```python
from build123d import *

# Parameters (mm, degrees)
SKETCH_W     = 12
SKETCH_H     = 9
SKETCH_R     = 1.7
PAD_DEPTH    = 2
SKETCH001_W  = 3.1
SKETCH001_H  = 4.7
PAD001_DEPTH = 2
SKETCH002_W  = 1.1
SKETCH002_H  = 5
POCKET_DEPTH = 4.001
CHAMFER_SIZE = 1.7


with BuildPart() as part:
    # Sketch → Pad (new body)
    with BuildSketch(Plane.XY):
        with Locations((-1.5, 0)):
            Rectangle(SKETCH_W, SKETCH_H)
        with Locations((-3, 0)):
            Circle(SKETCH_R, mode=Mode.SUBTRACT)
    extrude(amount=PAD_DEPTH)

    # Sketch001 → Pad001 (new body)
    with BuildSketch(Plane.XY.offset(2)):
        with Locations((1.75, 0)):
            Rectangle(SKETCH001_W, SKETCH001_H)
    extrude(amount=PAD001_DEPTH)

    # Sketch002 → Pocket (cut, through all)
    with BuildSketch(Plane.XY.offset(4)):
        with Locations((1.75, 4)):
            Rectangle(SKETCH002_W, SKETCH002_H)
        with Locations((1.75, -4)):
            Rectangle(SKETCH002_W, SKETCH002_H)
    extrude(amount=-POCKET_DEPTH, mode=Mode.SUBTRACT)

    # Chamfer
    chamfer_edges = [part.edges().sort_by_distance(p)[0] for p in [
        (-4.7, 0, 0),
    ]]
    chamfer(chamfer_edges, length=CHAMFER_SIZE)


solid = part.part
```
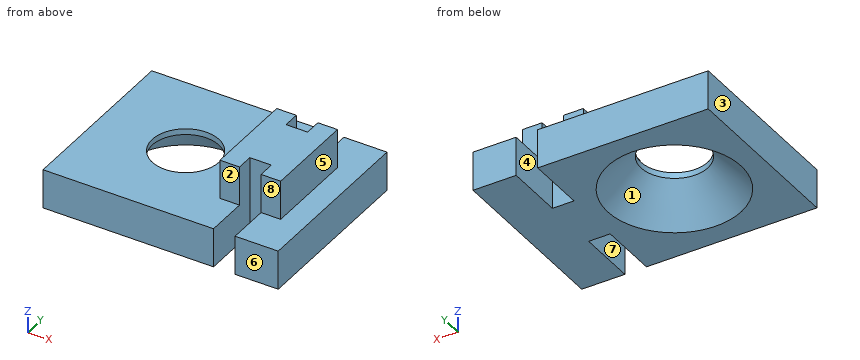
The model under review builds one solid part; all positions refer to its coordinate system, in mm. Face numbers are marked on the shaded views. A direction names the side the tool comes from. Coordinates: 2 decimals unless noted, no trailing zeros. Write each loop counter-clockwise with the first axis right and the second up, starting at its lowest first coordinate (ties: lowest second). Pieces come first, ordered by that corner, then holes. Notation, with made-up numbers: (60.25, -0.5) - (95.25, -0.5) arc R18 cw to (95.25, 14.5) - close; hole circle Ø11 at (-2, -14.5). An arc over 180 degrees is marked (long way). Write item = value, one per line.
(1) For P1, Ø0.5, axis at x = 0.5, z = 2.5, coming from the -Y side; P2, Ø4.5, axis at x = -4.5, y = -1.5, coming from the +Z side, all flat-tipped, find the tip position at first contact; note any pin that passes through.
Result sheet:
P1 = -2.35
P2 = 2
(2) Machinability: for the marked faces 4, 5, 6, 7 and 8, which of the approach directions +Z, -Z, +X, -X, +Y, -Y give a long, thin tool a straight path to every point of the face, cutting with its end or side? Answer none if there is none.
Result sheet:
face_4 = +Z, -Z, +Y
face_5 = +Z, +X, +Y, -Y
face_6 = +Z, -Z, +X, -X, -Y
face_7 = +Z, -Z, -Y
face_8 = +Z, +X, -X, -Y
(3) Consider section D-D, the plane x = 2.5. Give the boundary of the cut face in (y, z).
Result sheet:
outline = (-4.5, 0) - (4.5, 0) - (4.5, 2) - (2.35, 2) - (2.35, 4) - (-2.35, 4) - (-2.35, 2) - (-4.5, 2) - close
(4) For line 1 (X direction, y = 4, z = 0.8); line 2 (X direction, y = 2, z = 0.65); line 3 (X direction, y = 1.75, z = 0.3), list the stretches that pass through material, from the lowest coordinate up. Write a range as [from, to].
Result sheet:
line_1 = [-7.5, 1.2], [2.3, 4.5]
line_2 = [-7.5, -4.89], [-1.11, 1.2], [2.3, 4.5]
line_3 = [-7.5, -5.56], [-0.44, 1.2], [2.3, 4.5]
(5) Consider section B-B, the plane z = 0.9. Give the boundary of the cut face in (x, y).
Result sheet:
outline = (-7.5, -4.5) - (1.2, -4.5) - (1.2, -1.5) - (2.3, -1.5) - (2.3, -4.5) - (4.5, -4.5) - (4.5, 4.5) - (2.3, 4.5) - (2.3, 1.5) - (1.2, 1.5) - (1.2, 4.5) - (-7.5, 4.5) - close; hole circle Ø5 at (-3, 0)
(6) Consider section C-C, the plane y = 0. Give the boundary of the cut face in (x, z).
Result sheet:
outline = (-7.5, 0) - (-6.4, 0) - (-4.7, 1.7) - (-4.7, 2) - (-7.5, 2) - close; (-1.3, 1.7) - (0.4, 0) - (4.5, 0) - (4.5, 2) - (3.3, 2) - (3.3, 4) - (0.2, 4) - (0.2, 2) - (-1.3, 2) - close
(7) Consider section A-A, the plane x = -3. Give the boundary of the cut face in (y, z), then the cut area to 3 significant figures.
Result sheet:
outline = (-4.5, 0) - (-3.4, 0) - (-1.7, 1.7) - (-1.7, 2) - (-4.5, 2) - close; (1.7, 1.7) - (3.4, 0) - (4.5, 0) - (4.5, 2) - (1.7, 2) - close
area = 8.31 mm^2
(8) Mouldability with a two-part tool opening along X and no side actions: class the marked faces 1, 2 and 3 as pulls with the +X half, pulls with the -X half, needs draft (parallel to the pull), parting line crosses it, or undercut.
Result sheet:
face_1 = undercut
face_2 = needs draft
face_3 = pulls with the -X half
